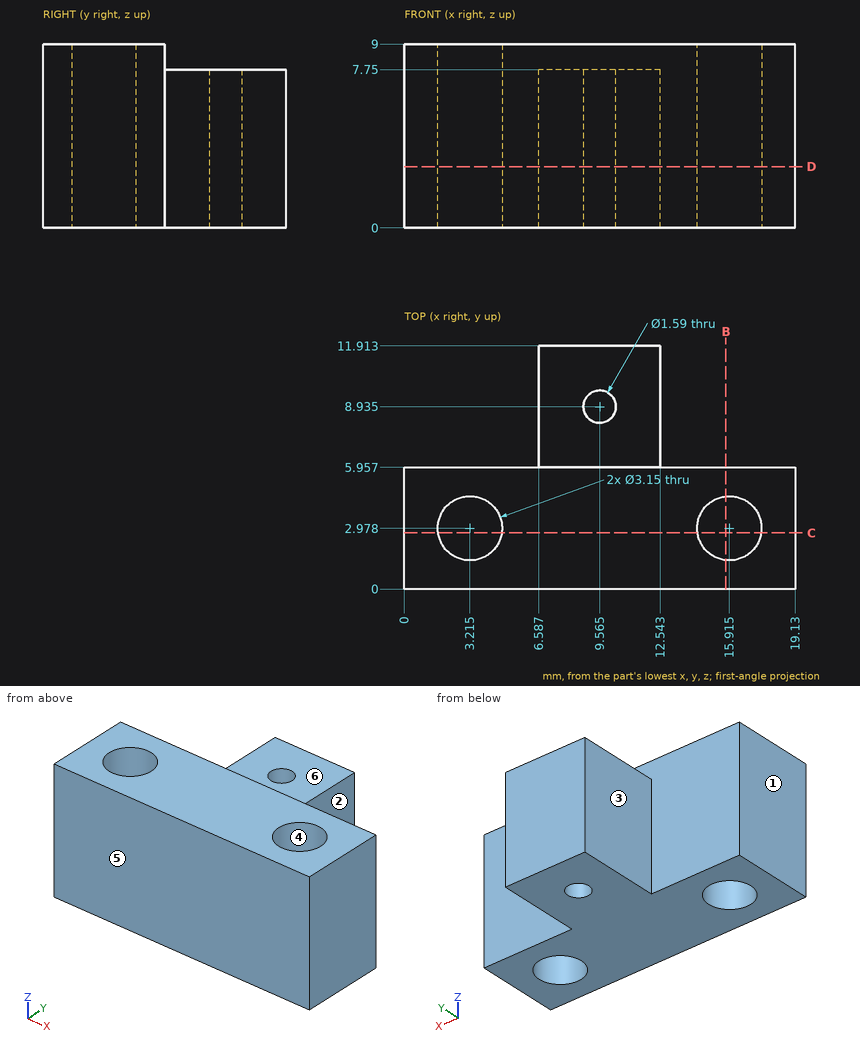
Geometry check sheet. Reference: drawing and pictorial views, mm from the part's lowest x, y, z. A direction names the side the tool comes from. Round coordinates to 2 decimals unless told otherwise and drop trailing zeros. Loops run counter-clockwise (first coordinate to the right, second up) from the corner with the lowest first, then second, coordinate; pieces in that order, holes last. Notation, with made-up numbers: (-38, 14.5) - (14, 14.5) arc R30 cw to (14, 38.5) - close; hole circle Ø8 at (27.5, -22). An arc over 180 degrees is marked (long way). Use a Markdown table: item, result. Add a question column.
1. Section check B-B, the plane x = 15.75. Record the boundary of the cut face in (y, z) (1 decimal).
2. Section check D-D, the plane z = 3. Give the number of separate pieces and of enclosed holes in the cut face, plus the area to 3 significant figures.
3. Section check C-C, the plane y = 2.75. Record the boundary of the cut face in (x, z), plus the area to 3 significant figures.
4. Release check for a two-part mould opening along Y. For the marked faces 4, 5 and 6 record: released by +Y, released by -Y, zero draft, split by the parting line, or undercut.
5. Gauge pin test, flat ends, axial feed: pin 1 (1.8 mm diameter, centred on y = 8.5, z = 5, fed in from +X); pin 2 (1.5 mm diameter, centred on y = 9, z = 2.5, fed in from -X); pin 3 (1.9 mm diameter, centred on x = 15.92, y = 2.98, fed in from +Z). Record the tip position at first contact, or that the pin passes through.
6. Access from +Z, -Z, +X, -X, +Y, -Y to the whole of each face (thin tool, end or side, straight path). Record for the marked faces 1, 2 and 3.
7. Thickness scan on probe 1 along Y at (x, z) = (16, 8.25) (1 decimal); probe 2 along Z at (x, y) = (8.75, 8); probe 3 along Y at (x, z) = (10, 0.5) (1 decimal). Record the ranges inside material, lowest first. Write a range as [from, to].
Checks:
| question | item | result |
|---|---|---|
| 1 | outline | (0, 0) - (1.4, 0) - (1.4, 9) - (0, 9) - close; (4.5, 0) - (6, 0) - (6, 9) - (4.5, 9) - close |
| 2 | separate pieces | 1 |
| 2 | enclosed holes | 3 |
| 2 | area | 132 mm^2 |
| 3 | outline | (0, 0) - (1.66, 0) - (1.66, 9) - (0, 9) - close; (4.77, 0) - (14.36, 0) - (14.36, 9) - (4.77, 9) - close; (17.47, 0) - (19.13, 0) - (19.13, 9) - (17.47, 9) - close |
| 3 | area | 116 mm^2 |
| 4 | face 4 | undercut |
| 4 | face 5 | released by -Y |
| 4 | face 6 | zero draft |
| 5 | pin 1 | stops at x = 12.54 |
| 5 | pin 2 | stops at x = 6.59 |
| 5 | pin 3 | passes through |
| 6 | face 1 | +Z, -Z, -X, +Y, -Y |
| 6 | face 2 | +Z, -Z, +X, +Y |
| 6 | face 3 | +Z, -Z, -X, +Y |
| 7 | probe 1 | y = [0, 1.4], [4.6, 6] |
| 7 | probe 2 | z = [0, 7.75] |
| 7 | probe 3 | y = [0, 8.3], [9.6, 11.9] |
